Here's the drawing with two shaded views (mm, measured from the low corner). I have some questions. Round coordinates to 2 decimals unless told otherwise and drop trailing zeros. Order: outer loops, then holes, each group sorted by start corner. A loop starts at its lowest first (then second) coordinate and runs counter-clockwise, first axis right, second up. Notation, with made-up numbers: (29, 38) -> (41, 38) arc R32 cw to (41, 70) -> close; hole circle Ø3 at (20.5, 58.5). An arc over 180 degrees is marked (long way). One line per question, with ' | ' between items.
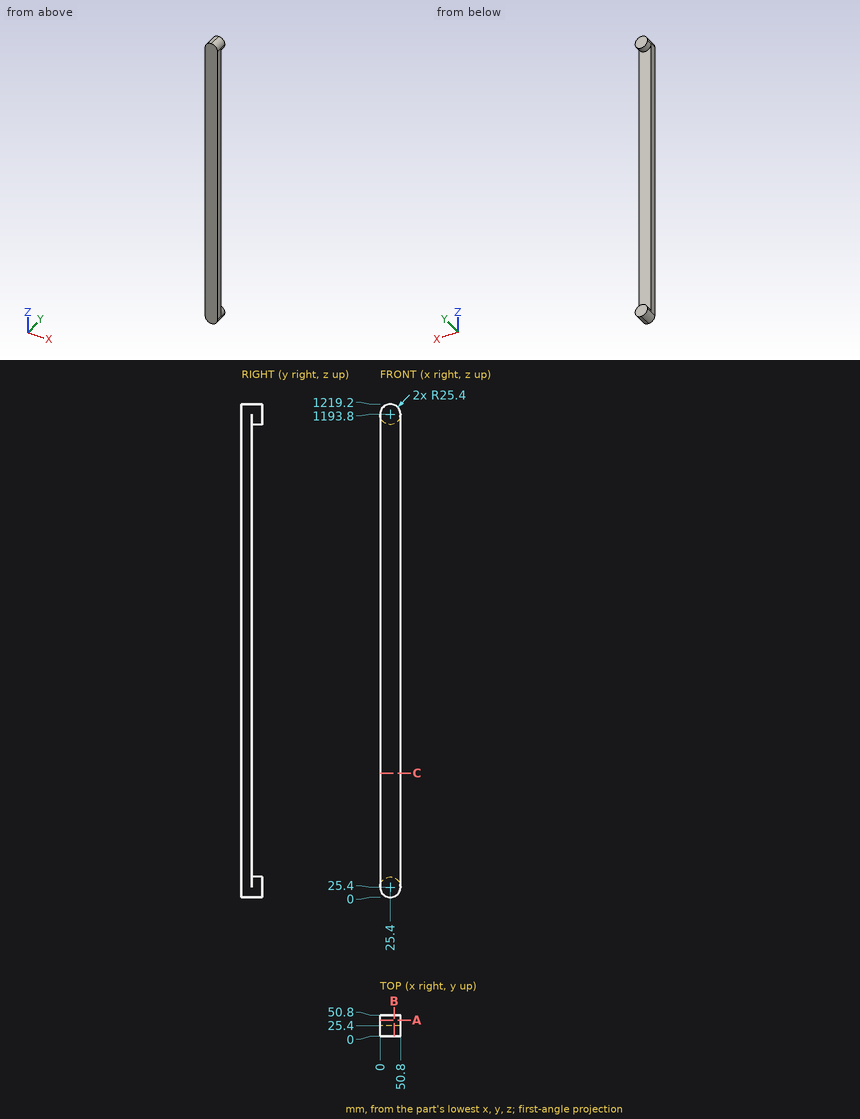
1. I'm going to push flat-ended pins straight in: pin 1 (10 mm diameter, centred on x = 41, z = 913, fed in from +Y); pin 2 (10 mm diameter, centred on x = 33, y = 30.5, fed in from +Z); pin 3 (10 mm diameter, centred on x = 31.5, y = 40.5, fed in from +Z). Where does each tip first touch, or does it pass through?
From the geometry:
pin 1: stops at y = 25.4 | pin 2: stops at z = 1219.07 | pin 3: stops at z = 1219.18
2. I want a section at C-C on z = 307. List the corners of the cut face in (x, y) for me, and give its area (3 significant figures).
From the geometry:
outline: (0, 0) -> (50.8, 0) -> (50.8, 25.4) -> (0, 25.4) -> close | area: 1,290 mm²
3. I want a section at A-A on y = 39.5. List the corners of the cut face in (x, z) for me.
From the geometry:
outline: circle Ø50.8 at (25.4, 25.4); circle Ø50.8 at (25.4, 1193.8)
4. I need wall thicknesses on probe 1 along Y at (x, z) = (35, 540); probe 2 along Z at (x, y) = (27, 3); probe 3 along Z at (x, y) = (24, 13.5). Which ranges of each line are inside material? Lowest first, please.
From the geometry:
probe 1: y = 0 to 25.4 | probe 2: z = 0.05 to 1219.15 | probe 3: z = 0.04 to 1219.16
5. I want a section at B-B on x = 35. List the corners of the cut face in (y, z) for me.
From the geometry:
outline: (0, 1.88) -> (50.8, 1.88) -> (50.8, 48.92) -> (25.4, 48.92) -> (25.4, 1170.28) -> (50.8, 1170.28) -> (50.8, 1217.32) -> (0, 1217.32) -> close
